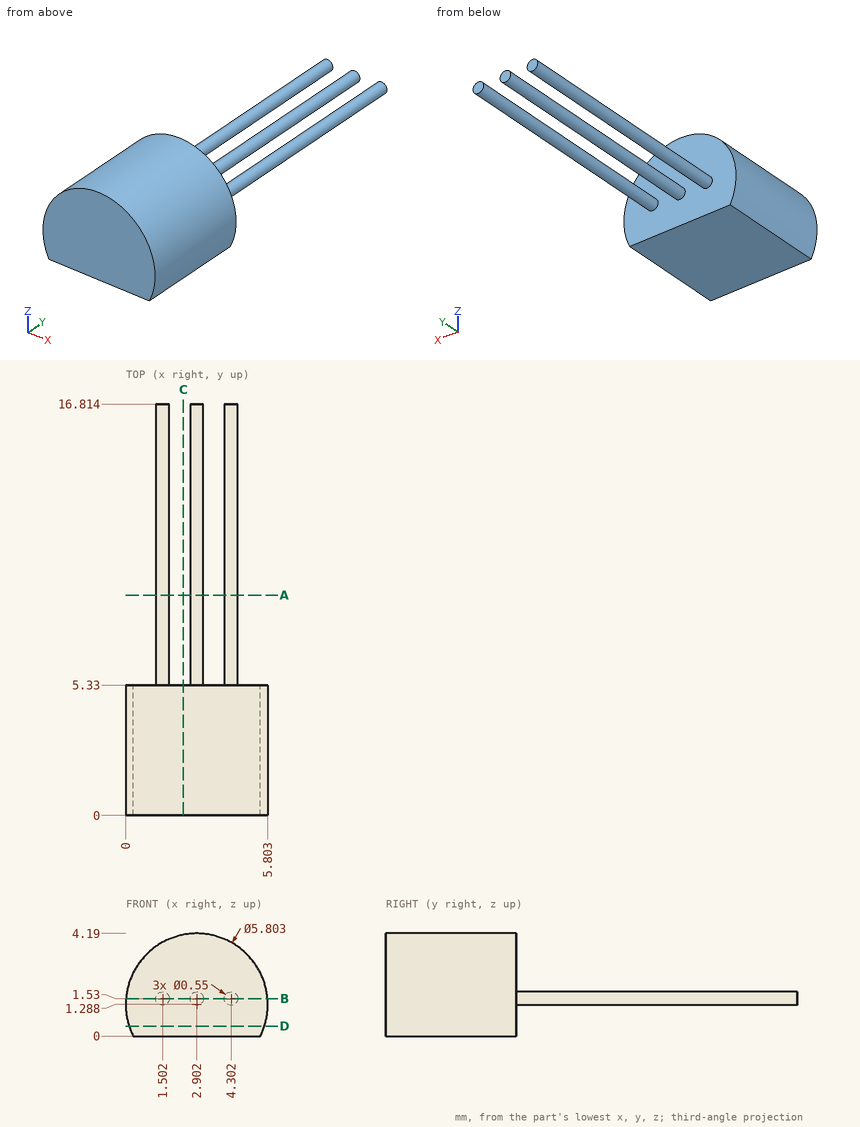
Here's the drawing with two shaded views (mm, measured from the low corner). I have some questions. Coordinates: 2 decimals unless noted, no trailing zeros. Loops run counter-clockwise (first coordinate to the right, second up) from the corner with the lowest first, then second, coordinate; pieces in that order, holes last. Notation, with made-up numbers: (-35, 72.5) - (-9, 72.5) arc R12 cw to (-9, 88.5) - close; hole circle Ø6 at (20, 37). An arc over 180 degrees is marked (long way). Answer as CSV lines item,"result". Start each with the question number.
1) I need wall thicknesses on line 1 (X direction, y = 9.75, z = 1.75) (1 decimal); line 2 (X direction, y = 11, z = 1.45) (1 decimal); line 3 (Y direction, x = 4.35, z = 0.3). Which ranges of each line are inside material? Lowest first, please. Write a range as from..to.
2) Suppose I cut it at D-D (z = 0.4). Please give me the cut outline in (x, y).
3) Suppose I cut it at A-A (y = 9). Count the separate pieces of the cut face and the enclosed holes in it.
4) For pin 1 (1 mm diameter, centred on x = 0.5, y = 11, fed in from +Z); pin 2 (1 mm diameter, centred on x = 3, z = 2.5, fed in from +Y), each with a flat end and sliding along its axis, tell me the tip position at first contact or that it passes through.
5) Suppose I cut it at C-C (x = 2.35). Please give me the cut outline in (y, z).
6) Suppose I cut it at B-B (z = 1.53). Please give me the cut outline in (x, y) (1 decimal).
Check result:
1,line 1,"x = 1.3..1.7, 2.7..3.1, 4.1..4.5"
1,line 2,"x = 1.2..1.8, 2.6..3.2, 4..4.6"
1,line 3,"y = 0..5.33"
2,outline,"(0.14, 0) - (5.66, 0) - (5.66, 5.33) - (0.14, 5.33) - close"
3,separate pieces,"3"
3,enclosed holes,"0"
4,pin 1,"passes through"
4,pin 2,"stops at y = 5.33"
5,outline,"(0, 0) - (5.33, 0) - (5.33, 4.14) - (0, 4.14) - close"
6,outline,"(0, 0) - (5.8, 0) - (5.8, 5.3) - (4.6, 5.3) - (4.6, 16.8) - (4, 16.8) - (4, 5.3) - (3.2, 5.3) - (3.2, 16.8) - (2.6, 16.8) - (2.6, 5.3) - (1.8, 5.3) - (1.8, 16.8) - (1.2, 16.8) - (1.2, 5.3) - (0, 5.3) - close"
